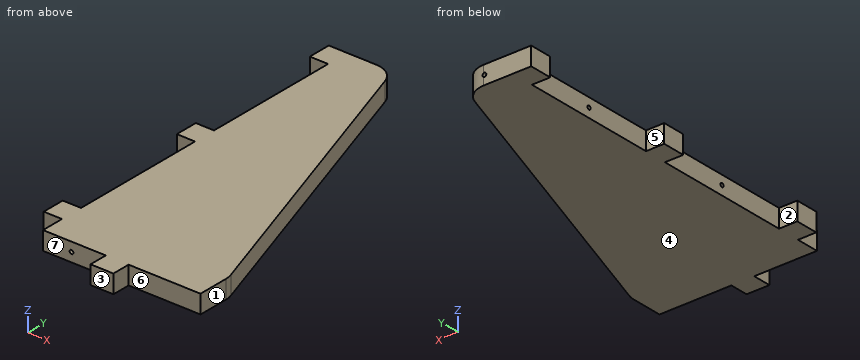
```python
from build123d import *

# Parameters (mm, degrees)
F1_DEPTH = 16
F2_W     = 16
F2_H     = 20
F2_W_2   = 20
F2_H_2   = 16
F3_DEPTH = 16
F4_R     = 20
F6_D     = 3.3
F6_DEPTH = 20
F6_TIP   = 0.9914200214
F8_D     = 3.3


with BuildPart() as f1:
    # F0 (on Top) → F1 (new body)
    with BuildSketch(Plane.XY):
        Polygon((0, 320), (0, 0), (138, 0), (138, 30), (40, 320), align=None)
    extrude(amount=F1_DEPTH)

    # F2 (on face) → F3 (join, through all)
    with BuildSketch(Plane.XY.offset(16)):
        with Locations((-8, 310)):
            Rectangle(F2_W, F2_H)
        with Locations((-8, 170)):
            Rectangle(F2_W, F2_H)
        with Locations((65, -8)):
            Rectangle(F2_W_2, F2_H_2)
        with Locations((-8, 30)):
            Rectangle(F2_W, F2_H)
    extrude(amount=-F3_DEPTH)

    # F4
    f4_edges = [f1.edges().sort_by_distance(p)[0] for p in [
        (40, 320, 8),
        (138, 30, 8),
    ]]
    fillet(f4_edges, radius=F4_R)

    # F6
    with Locations(Plane(origin=(0, 0, 0), x_dir=(0, -1, 0), z_dir=(-1, 0, 0))):
        with Locations((-240, 8), (-100, 8)):
            Hole(F6_D / 2, depth=F6_DEPTH)
            with Locations((0, 0, -(F6_DEPTH + F6_TIP / 2))):  # 118° drill point
                Cone(0, F6_D / 2, F6_TIP, mode=Mode.SUBTRACT)

    # F8 (through all)
    with Locations(Plane.XZ):
        with Locations((25, 8)):
            Hole(F8_D / 2)


solid = f1.part
```
Can you work these out from the model? Positions are in its coordinate system, mm. Face numbers are marked on the shaded views. A direction names the side the tool comes from. Coordinates: 2 decimals unless noted, no trailing zeros. Loops run counter-clockwise (first coordinate to the right, second up) from the corner with the lowest first, then second, coordinate; pieces in that order, holes last. Notation, with made-up numbers: M 13,87.25 L 38,87.25 A15 cw 38,93.25 Z; hole C -18.75,0 d4. An arc over 180 degrees is marked long. Put each result on its own line as item: value. Start each with the question number.
(1) I need wall thicknesses on probe 1 along Y at (x, z) = (8.25, 8); probe 2 along Z at (x, y) = (25, 122.5); probe 3 along Y at (x, z) = (1, 15). Which ranges of each line are inside material? Lowest first, please.
(2) We'd pull the mould along Y, two halves only. Please class the marked faces 1, 2 and 3: +Y half, -Y half, draft (parallel to the pull), parting line (faces both ways), or undercut.
(3) Imagine slicing it at B-B on x = 71. List the corners of the cut face in (y, z) for me.
(4) Imagine slicing it at D-D on x = 113. List the corners of the cut face in (y, z) for me, and give its area (3 significant figures).
(5) Imagine slicing it at A-A on y = 271.5. List the corners of the cut face in (x, z) for me, and give its area (3 significant figures).
(6) Imagine slicing it at C-C on y = 222.5. List the corners of the cut face in (x, z) for me, and give its area (3 significant figures).
(7) Will these pins go through, and if not, where does the flat tip stop? pin 1 Ø4 at (y, z) = (49.5, 8.5) entering from +X; pin 2 Ø8 at (x, z) = (-9, 10) entering from -Y; pin 3 Ø6 at (y, z) = (48.5, 12.5) entering from -X.
(8) Which directions (+Z, -Z, +X, -X, +Y, -Y) give clear straight access to the entire face, cutting with the end or side of a thin tool? Please do the marked faces 4, 5, 6 and 7.
Worked answers:
1. probe 1: y = 0 to 98.35, 101.65 to 238.35, 241.65 to 320
1. probe 2: z = 0 to 6.35, 9.65 to 16
1. probe 3: y = 0 to 320
2. face 1: draft
2. face 2: undercut
2. face 3: -Y half
3. outline: M -16,0 L 228.27,0 L 228.27,16 L -16,16 Z
4. outline: M 0,0 L 103.98,0 L 103.98,16 L 0,16 Z
4. area: 1,660 mm2
5. outline: M 0,0 L 56.39,0 L 56.39,16 L 0,16 Z; hole C 25,8 d3.3
5. area: 894 mm2
6. outline: M 0,0 L 72.95,0 L 72.95,16 L 0,16 Z; hole C 25,8 d3.3
6. area: 1,160 mm2
7. pin 1: stops at x = 132.09
7. pin 2: stops at y = 20
7. pin 3: stops at x = 0
8. face 4: -Z, +X, -X, +Y, -Y
8. face 5: +Z, -Z, -X
8. face 6: +Z, -Z, +X, -Y
8. face 7: +Z, -Z, -X, -Y
